from build123d import *

# Parameters (mm, degrees)
SKETCH1_R           = 22
SKETCH1_R_2         = 12.5
BOSS_EXTRUDE1_DEPTH = 15
CHAMFER1_SIZE       = 1
CHAMFER2_SIZE       = 5
CHAMFER2_SIZE2      = 10
CHAMFER3_SIZE       = 10
CHAMFER3_SIZE2      = 5


with BuildPart() as part:
    # Sketch1 → Boss-Extrude1 (new, symmetric)
    with BuildSketch(Plane.XY):
        Circle(SKETCH1_R)
        Circle(SKETCH1_R_2, mode=Mode.SUBTRACT)
    extrude(amount=BOSS_EXTRUDE1_DEPTH, both=True)

    # Chamfer1
    chamfer1_edges = [part.edges().sort_by_distance(p)[0] for p in [
        (-22, 0, -15),
        (-22, 0, 15),
    ]]
    chamfer(chamfer1_edges, length=CHAMFER1_SIZE)

    # Chamfer2
    chamfer2_edges = [part.edges().sort_by_distance(p)[0] for p in [
        (-12.5, 0, 15),
    ]]
    chamfer2_side = [part.faces().sort_by_distance(p)[0] for p in [
        (-20.406030304, 0, 15),
    ]]
    chamfer(chamfer2_edges, length=CHAMFER2_SIZE, length2=CHAMFER2_SIZE2, reference=chamfer2_side[0])

    # Chamfer3
    chamfer3_edges = [part.edges().sort_by_distance(p)[0] for p in [
        (-12.5, 0, -15),
    ]]
    chamfer3_side = [part.faces().sort_by_distance(p)[0] for p in [
        (-12.5, 0, -5),
    ]]
    chamfer(chamfer3_edges, length=CHAMFER3_SIZE, length2=CHAMFER3_SIZE2, reference=chamfer3_side[0])

    # Sketch2 → Cut-Revolve1 (revolve, cut)
    with BuildSketch(Plane(origin=(-103.136389545, -329.994936254, 0), x_dir=(-1, 0, 0), z_dir=(0, 0, 1)), mode=Mode.PRIVATE) as cut_revolve1_sk:
        Polygon((-103.136389545, -304.994936254), (-103.136389545, -316.494936254), (-96.496861449, -304.994936254), align=None)
    cut_revolve1 = revolve(cut_revolve1_sk.sketch.rotate(Axis((0, -25, 0), (0, 1, 0)), 270), axis=Axis((0, -25, 0), (0, 1, 0)), mode=Mode.SUBTRACT)

    # Mirror3: Cut-Revolve1 across plane
    add(cut_revolve1.mirror(Plane.ZX), mode=Mode.SUBTRACT)


solid = part.part
The listing builds one solid part. Answer for the finished solid, in the listing's coordinates (mm). Round coordinates to 2 decimals unless told otherwise and drop trailing zeros. Write each loop counter-clockwise with the first axis right and the second up, starting at its lowest first coordinate (ties: lowest second). Pieces come first, ordered by that corner, then holes. Notation, with made-up numbers: M 11,1.25 L 63,1.25 A19 cw 63,20.25 Z; hole C 81,52.25 d8. An arc over 180 degrees is marked long. Write each question's results on one line, items separated by ' | '. Start each with the question number.
Item 1: A cutting plane is placed at A-A on y = 0. Write down the section's boundary in (x, z), and give its area (3 significant figures).
Item 2: A cutting plane is placed at C-C on z = 9. Write down the section's boundary in (x, y), and give its area (3 significant figures).
Item 3: Straight lines are drawn through the part: L1, parallel to X at y = 4, z = -11; L2, parallel to X at y = -13.5, z = -10; L3, parallel to Y at x = 5, z = -12. For each, find the intervals that lie inside material, in ascending order. Write a range as [from, to].
Item 4: A cutting plane is placed at B-B on z = -10. Write down the section's boundary in (x, y), and give its area (3 significant figures).
Item 5: For a pull along X with two mould halves and no side action, classify faces 1 (the face through (-10.112, -7.754, 5.486)), 2 (the face through (-8, 16, 15)), 3 (the face through (-4.769, -21.477, 0.196)) as pulls with the +X half, pulls with the -X half, needs draft (parallel to the pull), parting line crosses it, or undercut.
Item 6: Flat-ended cylindrical pins translate along their axes: pin 1 Ø2 at (x, y) = (1, -16) entering from +Z; pin 2 Ø1 at (y, z) = (-14, 5.5) entering from +X; pin 3 Ø1.5 at (x, z) = (7, -5) entering from -Y; pin 4 Ø15 at (x, y) = (0, 0) entering from +Z. Find the tip coordinate at first contact, or state that the pin passes through.
Check sheet entries:
1) outline: M -22,-14 L -21,-15 L -17.5,-15 L -12.5,-5 L -12.5,5 L -17.5,15 L -21,15 L -22,14 Z; M 12.5,-5 L 17.5,-15 L 21,-15 L 22,-14 L 22,14 L 21,15 L 17.5,15 L 12.5,5 Z | area: 468 mm²
2) outline: C 0,0 d44; hole C 0,0 d29 | area: 860 mm²
3) L1: [-21.63, -14.97], [14.97, 21.63] | L2: [-17.37, -6.54], [6.54, 17.37] | L3: [-21.42, -15.2], [15.2, 21.42]
4) outline: C 0,0 d44; hole C 0,0 d30 | area: 814 mm²
5) face 1: undercut | face 2: needs draft | face 3: parting line crosses it
6) pin 1: z = 14.06 | pin 2: x = 17.37 | pin 3: y = -21.09 | pin 4: through
